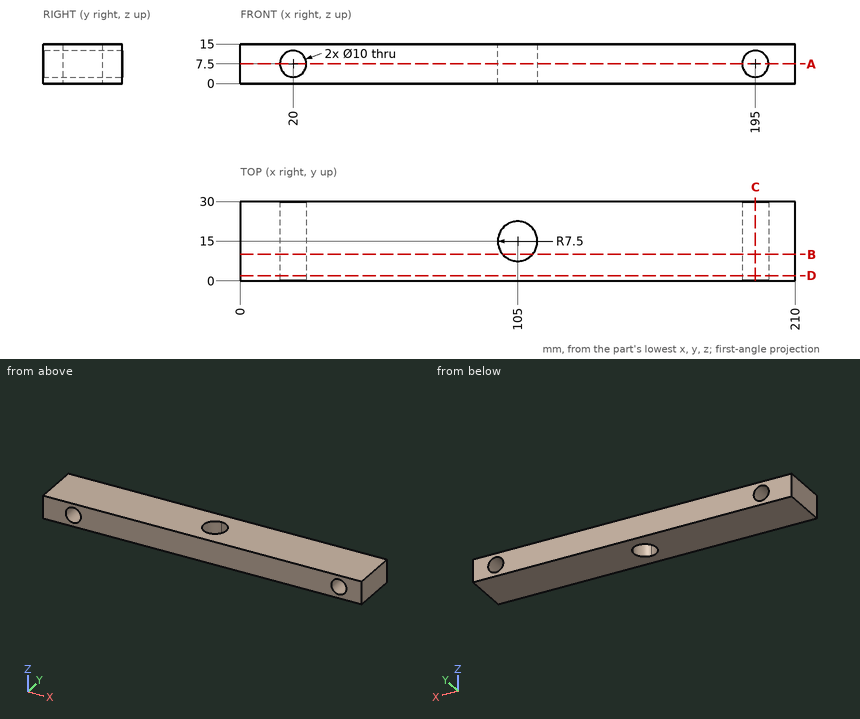
Source: three-view drawing plus pictorial views. Frame: mm from the lowest corner of the part. Coordinates: 2 decimals unless noted, no trailing zeros. Loops run counter-clockwise (first coordinate to the right, second up) from the corner with the lowest first, then second, coordinate; pieces in that order, holes last. Notation, with made-up numbers: (5.25, 47.25) - (61.25, 47.25) arc R25 cw to (61.25, 74.25) - close; hole circle Ø3 at (-8, 75.5). An arc over 180 degrees is marked (long way). One line per item, written item: value. Start each with the question number.
1. Ray query, L1, parallel to X at y = 24.25, z = 7.5; L2, parallel to X at y = 3.25, z = 9.75; L3, parallel to X at y = 8.25, z = 10.5. Return the intervals inside material, ascending.
2. Section B-B (y = 10). Return the cut outline in (x, z).
3. Section D-D (y = 2). Return the cut outline in (x, z), and give its area (3 significant figures).
4. Section A-A (z = 7.5). Return the cut outline in (x, y), and give its area (3 significant figures).
5. Section C-C (x = 195). Return the cut outline in (y, z), and give its area (3 significant figures).
Verdict:
1. L1: x = 0 to 15, 25 to 190, 200 to 210
1. L2: x = 0 to 15.53, 24.47 to 190.53, 199.47 to 210
1. L3: x = 0 to 16, 24 to 101.73, 108.27 to 191, 199 to 210
2. outline: (0, 0) - (99.41, 0) - (99.41, 15) - (0, 15) - close; (110.59, 0) - (210, 0) - (210, 15) - (110.59, 15) - close; hole circle Ø10 at (20, 7.5); hole circle Ø10 at (195, 7.5)
3. outline: (0, 0) - (210, 0) - (210, 15) - (0, 15) - close; hole circle Ø10 at (20, 7.5); hole circle Ø10 at (195, 7.5)
3. area: 2,990 mm2
4. outline: (0, 0) - (15, 0) - (15, 30) - (0, 30) - close; (25, 0) - (190, 0) - (190, 30) - (25, 30) - close; (200, 0) - (210, 0) - (210, 30) - (200, 30) - close; hole circle Ø15 at (105, 15)
4. area: 5,520 mm2
5. outline: (0, 0) - (30, 0) - (30, 2.5) - (0, 2.5) - close; (0, 12.5) - (30, 12.5) - (30, 15) - (0, 15) - close
5. area: 150 mm2
